```python
from build123d import *

# Parameters (mm, degrees)
SKETCH1_W                  = 80
SKETCH1_H                  = 80
PCB_DEPTH                  = 2
SKETCH2_R                  = 1.8
ATTACHMENT_HOLES_DEPTH     = 3
LPATTERN1_COUNT            = 2
LPATTERN1_PITCH            = 70
LPATTERN1_COUNT_DIR2       = 2
LPATTERN1_PITCH_DIR2       = 70
SKETCH3_W                  = 57
SKETCH3_H                  = 30
COMMS_CHIP_DEPTH           = 12.8
SKETCH4_R                  = 1.115
COMM_CHIP_ATTACHMENT_DEPTH = 15.8
LPATTERN2_COUNT            = 2
LPATTERN2_PITCH            = 25
SKETCH5_W                  = 34
SKETCH5_H                  = 24
ARDUCAMMINI_DEPTH          = 5
SKETCH8_R                  = 5
LENS_APPROXIMATE_DEPTH     = 8
SKETCH6_W                  = 25.4
SKETCH6_H                  = 31.85
SD_CARD_DEPTH              = 3.75
SKETCH7_R                  = 3.95
ANTENNA_DEPTH              = 300


with BuildPart() as part:
    # Sketch1 → PCB (new body)
    with BuildSketch(Plane(origin=(0, 0, 0), x_dir=(1, 0, 0), z_dir=(0, 1, 0))):
        with Locations((40, 40)):
            Rectangle(SKETCH1_W, SKETCH1_H)
    extrude(amount=PCB_DEPTH)

    # Sketch2 → Attachment Holes (cut, through all)
    with BuildSketch(Plane(origin=(0, 2, 0), x_dir=(1, 0, 0), z_dir=(0, 1, 0))):
        with Locations((5, 75)):
            Circle(SKETCH2_R)
    attachment_holes = extrude(amount=-ATTACHMENT_HOLES_DEPTH, mode=Mode.SUBTRACT)

    # LPattern1: Attachment Holes 2 × 2
    with Locations(*[(i * LPATTERN1_PITCH, 0, j * LPATTERN1_PITCH_DIR2) for i in range(LPATTERN1_COUNT) for j in range(LPATTERN1_COUNT_DIR2) if (i, j) != (0, 0)]):
        add(attachment_holes, mode=Mode.SUBTRACT)

    # Sketch3 → Comms Chip (add)
    with BuildSketch(Plane(origin=(0, 0, 0), x_dir=(1, 0, 0), z_dir=(0, 1, 0))):
        with Locations((40, 60)):
            Rectangle(SKETCH3_W, SKETCH3_H)
    extrude(amount=-COMMS_CHIP_DEPTH)

    # Sketch4 → Comm chip attachment (cut, through all)
    with BuildSketch(Plane(origin=(0, -12.8, 0), x_dir=(-1, 0, 0), z_dir=(0, -1, 0))):
        with Locations((-4, 77.5)):
            Circle(SKETCH4_R)
    comm_chip_attachment = extrude(amount=-COMM_CHIP_ATTACHMENT_DEPTH, mode=Mode.SUBTRACT)

    # LPattern2: Comm chip attachment ×2
    with Locations(*[(0, 0, i * LPATTERN2_PITCH) for i in range(1, LPATTERN2_COUNT)]):
        add(comm_chip_attachment, mode=Mode.SUBTRACT)

    # Sketch5 → ArducamMini (add)
    with BuildSketch(Plane(origin=(0, 2, 0), x_dir=(1, 0, 0), z_dir=(0, 1, 0))):
        with Locations((25, 20)):
            Rectangle(SKETCH5_W, SKETCH5_H)
    extrude(amount=ARDUCAMMINI_DEPTH)

    # Sketch8 → Lens, approximate (add)
    with BuildSketch(Plane(origin=(0, 7, 0), x_dir=(1, 0, 0), z_dir=(0, 1, 0))):
        with Locations((18, 20)):
            Circle(SKETCH8_R)
    extrude(amount=LENS_APPROXIMATE_DEPTH)

    # Sketch6 → SD Card (add)
    with BuildSketch(Plane(origin=(0, 2, 0), x_dir=(1, 0, 0), z_dir=(0, 1, 0))):
        with Locations((59.3, 23.925)):
            Rectangle(SKETCH6_W, SKETCH6_H)
    extrude(amount=SD_CARD_DEPTH)

    # Sketch7 → Antenna (add)
    with BuildSketch(Plane(origin=(68.5, -53.7, 0), x_dir=(0, 1, 0), z_dir=(-1, 0, 0))):
        with Locations((47.9, 53)):
            Circle(SKETCH7_R)
    extrude(amount=-ANTENNA_DEPTH)


solid = part.part
```
Read the model definition and answer for the solid it produces. Units are mm, in the model's axes. A direction names the side the tool comes from. Round coordinates to 2 decimals unless told otherwise and drop trailing zeros. Write each loop counter-clockwise with the first axis right and the second up, starting at its lowest first coordinate (ties: lowest second). Pieces come first, ordered by that corner, then holes. Notation, with made-up numbers: (38.25, 70.5) -> (67.25, 70.5) arc R31 cw to (67.25, 100.5) -> close; hole circle Ø8 at (-25, 78.5). An arc over 180 degrees is marked (long way). Answer in a Markdown table with one row per item. Add a question column.
1) Find section B-B, the plane x = 165.5. Determine the outline of the cut face in (y, z), and give its area (3 significant figures).
2) Consider line 1 (X direction, y = 1.5, z = -5); line 2 (Z direction, x = 75, y = 1.15); line 3 (Z direction, x = 4, y = 1.25) (3 decimals). Determine where each line is inside the solid, lowest interval first.
3) Given P1, Ø7.5, axis at x = 61, z = -16.5, coming from the +Y side; P2, Ø3, axis at y = 11.5, z = -15.5, coming from the -X side; P3, Ø5, axis at y = 7, z = -27.5, coming from the +X side, each flat-ended and moving along its own axis, determine where each tip first touches the part or whether it passes through.
4) Find section A-A, the plane x = 18. Determine the outline of the cut face in (y, z).
5) Which of the six approach directions +Z, -Z, +X, -X, +Y, -Y give full straight-line access (tool end or side, diameter ignored) to faces 1 (the face through (216.4, -6.314, -56.916)), 2 (the face through (59, 5.75, -24)), 3 (the face through (40, -6, -45)), 4 (the face through (40, -6, -75))?
Findings below:
| question | item | result |
|---|---|---|
| 1 | outline | circle Ø7.9 at (-5.8, -53) |
| 1 | area | 49.0 mm² |
| 2 | line 1 | 0 to 3.2, 6.8 to 73.2, 76.8 to 80 |
| 2 | line 2 | -80 to -76.8, -73.2 to -6.8, -3.2 to 0 |
| 2 | line 3 | -80 to -78.615, -73.503 to -53.615, -51.385 to -6.497, -3.503 to 0 |
| 3 | P1 | y = 5.75 |
| 3 | P2 | x = 14 |
| 3 | P3 | x = 72 |
| 4 | outline | (-12.8, -75) -> (0, -75) -> (0, -80) -> (2, -80) -> (2, -32) -> (7, -32) -> (7, -25) -> (15, -25) -> (15, -15) -> (7, -15) -> (7, -8) -> (2, -8) -> (2, 0) -> (0, 0) -> (0, -45) -> (-12.8, -45) -> close |
| 5 | face 1 | +X |
| 5 | face 2 | +Z, -Z, +X, +Y |
| 5 | face 3 | +Z, +X, -X, -Y |
| 5 | face 4 | -Z, +X, -X, -Y |
